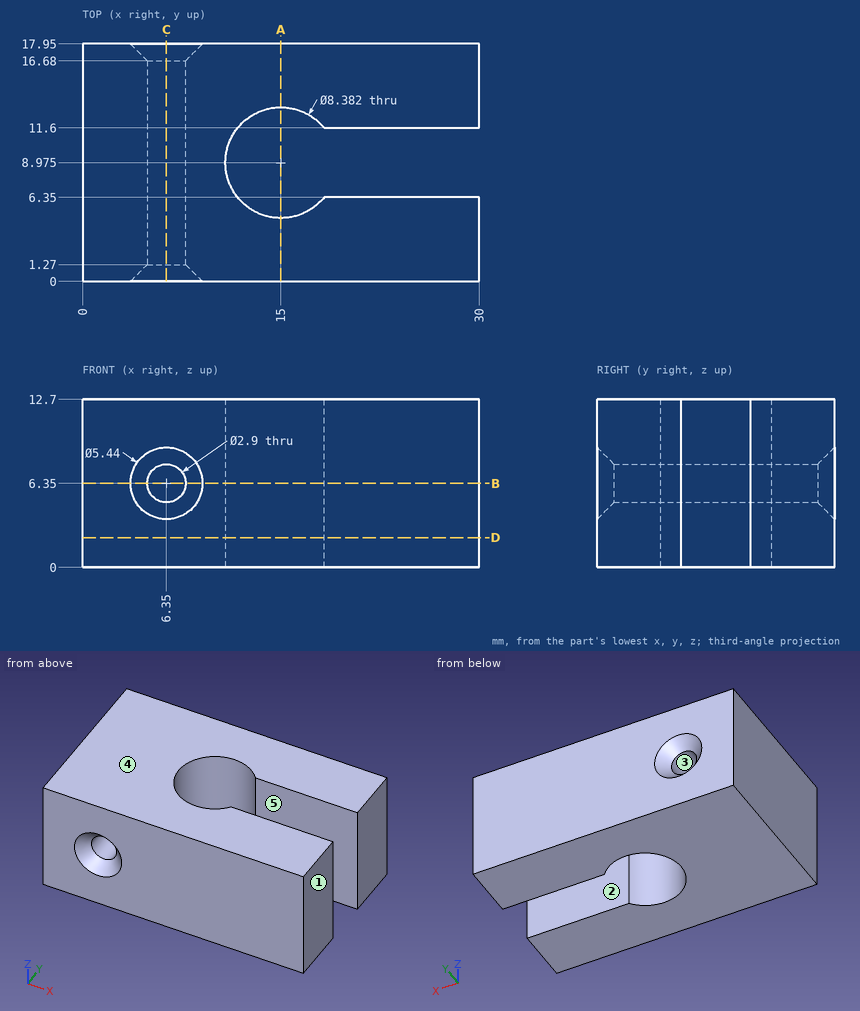
Study the drawing (mm; zero at the part's minimum x, y, z) and answer. A direction names the side the tool comes from. Give positions to 0.01 mm unless a question says otherwise; leave off trailing zeros. Order: outer loops, then holes, each group sorted by start corner. A loop starts at its lowest first (then second) coordinate and runs counter-clockwise, first axis right, second up. Notation, with made-up numbers: (-25.5, 23.5) -> (-9.5, 23.5) arc R10 cw to (-9.5, 35.5) -> close; hole circle Ø11 at (67, 48). An arc over 180 degrees is marked (long way). Write item = value, one per line.
1. A cutting plane is placed at A-A, the plane x = 15. Write down the section's boundary in (y, z).
Numbers:
outline = (0, 0) -> (4.78, 0) -> (4.78, 12.7) -> (0, 12.7) -> close; (13.17, 0) -> (17.95, 0) -> (17.95, 12.7) -> (13.17, 12.7) -> close
2. Straight lines are drawn through the part: line 1 along Y through (x, z) = (25, 7); line 2 along Y through (x, z) = (15, 3); line 3 along X through (y, z) = (5.75, 6). For each, find the intervals that lie inside material, in ascending order.
Numbers:
line_1 = 0 to 6.35, 11.6 to 17.95
line_2 = 0 to 4.78, 13.17 to 17.95
line_3 = 0 to 4.94, 7.76 to 12.32, 17.68 to 30
3. A cutting plane is placed at B-B, the plane z = 6.35. Write down the section's boundary in (x, y) (3 decimals).
Numbers:
outline = (0, 0) -> (3.63, 0) -> (4.9, 1.27) -> (4.9, 16.68) -> (3.63, 17.95) -> (0, 17.95) -> close; (7.8, 1.27) -> (9.07, 0) -> (30, 0) -> (30, 6.35) -> (18.267, 6.35) arc R4.191 cw (long way) to (18.267, 11.6) -> (30, 11.6) -> (30, 17.95) -> (9.07, 17.95) -> (7.8, 16.68) -> close
4. A cutting plane is placed at C-C, the plane x = 6.35. Write down the section's boundary in (y, z).
Numbers:
outline = (0, 0) -> (17.95, 0) -> (17.95, 3.63) -> (16.68, 4.9) -> (1.27, 4.9) -> (0, 3.63) -> close; (0, 9.07) -> (1.27, 7.8) -> (16.68, 7.8) -> (17.95, 9.07) -> (17.95, 12.7) -> (0, 12.7) -> close
5. The mould has two halves that part along X. Classify the marked faces 1, 2 and 3: +X half, -X half, draft (parallel to the pull), parting line (faces both ways), or undercut.
Numbers:
face_1 = +X half
face_2 = draft
face_3 = undercut
6. For the marked faces 4 and 5, determine the directions among +Z, -Z, +X, -X, +Y, -Y from which every point of the face is accessible in a straight line to the end or side of a thin tool.
Numbers:
face_4 = +Z, +X, -X, +Y, -Y
face_5 = +Z, -Z, +X
7. A cutting plane is placed at D-D, the plane z = 2.25. Write down the section's boundary in (x, y) (3 decimals).
Numbers:
outline = (0, 0) -> (30, 0) -> (30, 6.35) -> (18.267, 6.35) arc R4.191 cw (long way) to (18.267, 11.6) -> (30, 11.6) -> (30, 17.95) -> (0, 17.95) -> close
